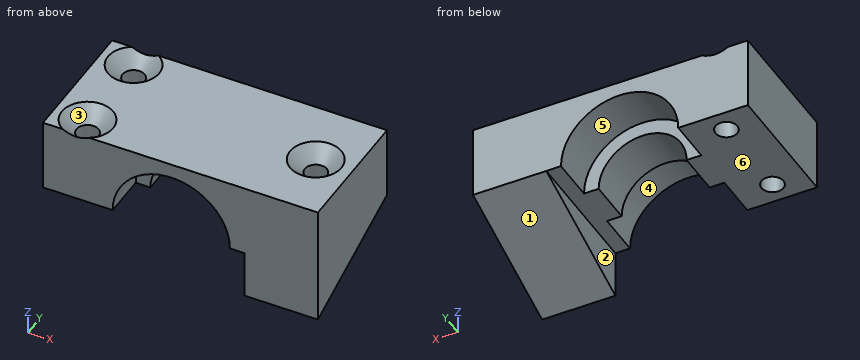
Autodesk Inventor part; units mm, degrees
ref_plane "YZ Plane" through (0, 0, 0) normal (1, 0, 0) x (0, 1, 0)
ref_plane "XZ Plane" through (0, 0, 0) normal (0, 1, 0) x (-1, 0, 0)
ref_plane "XY Plane" through (0, 0, 0) normal (0, 0, 1) x (1, 0, 0)
sketch "Sketch1" plane through (0, 0, 0) normal (0, 0, 1) x (1, 0, 0)
  line L0 (-13.216, 7.0679) -> (17.784, 7.0679) construction
  line L1 (17.784, 7.0679) -> (17.784, -7.9321) construction
  line L2 (17.784, -7.9321) -> (-13.216, -7.9321) construction
  line L3 (-13.216, -7.9321) -> (-13.216, 7.0679) construction
  circle A0 centre (-11.716, 5.5679) radius 1.5
  circle A1 centre (-11.716, -6.4321) radius 1.5
  circle A2 centre (16.284, -0.4321) radius 1.5
  line L4 (-16.216, 8.5679) -> (21.284, 8.5679)
  line L5 (21.284, 8.5679) -> (21.284, -9.4321)
  line L6 (21.284, -9.4321) -> (-16.216, -9.4321)
  line L7 (-16.216, -9.4321) -> (-16.216, 8.5679)
  point P0 (0, 0)
  dimension "d0" = 28
  dimension "d1" = 6
  dimension "d2" = 6
  dimension "d3" = 3
  dimension "d4" = 3
  dimension "d5" = 3
  dimension "d10" = 4.5
  dimension "d11" = 3
  dimension "d13" = 1.5
  dimension "d34" = 5
extrude "Extrusion1" add sketch "Sketch1" along normal blind 10
sketch "Sketch3" plane through (-16.216, -9.4321, 10) normal (0, -1, 0) x (1, 0, 0)
  line L0 (37.5, -10) -> (0, -10)
  circle A0 centre (17.5, -10) radius 6 construction
  line L1 (23.5, -10) -> (23.5, -2.9049) construction
  circle A1 centre (17.5, -10) radius 8
  line L2 (0, -10) -> (0, 0)
  line L3 (9.5, -10) -> (9.5, -3.6397) construction
  point P0 (27.5, -10)
  point P1 (16.216, -10)
  dimension "d19" = 12
  dimension "d21" = 16
  dimension "d30" = 9.5
extrude "Extrusion3" cut sketch "Sketch3" against normal blind 6
sketch "Sketch4" plane through (-16.216, -3.4321, 10) normal (0, -1, 0) x (1, 0, 0)
  arc A0 (25.5, -10) -> (9.5, -10) centre (17.5, -10) ccw
  circle A1 centre (17.5, -10) radius 6
  point P0 (16.216, -10)
  dimension "d24" = 12
extrude "Extrusion4" cut sketch "Sketch4" against normal blind 6
sketch "Sketch5" plane through (-16.216, 2.5679, 10) normal (0, -1, 0) x (1, 0, 0)
  arc A0 (23.5, -10) -> (11.5, -10) centre (17.5, -10) ccw
  circle A1 centre (17.5, -10) radius 8
  point P0 (16.216, -10)
  dimension "d27" = 16
extrude "Extrusion5" cut sketch "Sketch5" against normal blind 19.5
sketch "Sketch6" plane through (21.284, -9.4321, 0) normal (1, 0, 0) x (0, 0, -1)
  line L0 (0, 18) -> (0, 0)
  line L1 (0, 18) -> (-10, 18)
  line L2 (0, 0) -> (-10, 0)
  line L3 (0, 18) -> (6.5515, 0)
  line L4 (0, 18) -> (12.9005, 18) construction
  line L5 (0, 0) -> (6.5515, 0)
  point P0 (0, 9.4321)
  dimension "d31" = 70
extrude "Extrusion6" add sketch "Sketch6" against normal blind 10
chamfer "Chamfer1" distance 2 angle 45 3 edges at (-13.216, 5.5679, 10) (-13.216, -6.4321, 10) (14.784, -0.4321, 10)
equation "\"d4\" = d3"
equation "\"d5\" = d3"
properties part number "Lukker" material "PLA Plastic"
Can you work these out from the model? Positions are in its coordinate system, mm. Face numbers are marked on the shaded views. A direction names the side the tool comes from. Give positions to 0.01 mm unless a question says otherwise; leave off trailing zeros. Order: outer loops, then holes, each group sorted by start corner. A loop starts at its lowest first (then second) coordinate and runs counter-clockwise, first axis right, second up. Notation, with made-up numbers: M 53.25,69 L 102.25,69 A26 ccw 102.25,89 Z; hole C -12.75,21 d4. An arc over 180 degrees is marked long. Use a Markdown table: item, result. Add a question column.
Item 1: Suppose I cut it at C-C (z = -3.75). List the corners of the cut face in (x, y) for me.
Item 2: If I drill on L1, parallel to X at y = -0.5, z = 6.25; L2, parallel to X at y = -7.75, z = 3.75; L3, parallel to X at y = 0.5, z = -1.25, over which ranges is the centre line in solid material (lowest first)? Write a range as [from, to].
Item 3: For the marked faces 4, 5 and 6, which set-ups out of +Z, -Z, +X, -X, +Y, -Y let a thin tool reach every point of the face, with its end or its side?
Item 4: Will these pins go through, and if not, where does the flat tip stop? pin 1 (10 mm diameter, centred on x = -10, y = -4.5, fed in from -Z); pin 2 (5 mm diameter, centred on x = 16.28, y = -0.43, fed in from +Z); pin 3 (9 mm diameter, centred on x = 2.5, z = 2.5, fed in from -Y).
Item 5: Suppose I cut it at B-B (x = 2.5). List the corners of the cut face in (y, z) for me.
Item 6: Suppose I cut it at D-D (x = -3). List the corners of the cut face in (y, z) for me, then the cut area to 3 significant figures.
Item 7: We'd pull the mould along X, two halves only. Please class the marked faces 1, 2 and 3: +X half, -X half, draft (parallel to the pull), parting line (faces both ways), or undercut.
Item 8: Suppose I cut it at A-A (z = 2). List the corners of the cut face in (x, y) for me.
Answer sheet:
| question | item | result |
|---|---|---|
| 1 | outline | M 11.28,-9.43 L 21.28,-9.43 L 21.28,-1.74 L 11.28,-1.74 Z |
| 2 | L1 | x = [-16.22, 14.79], [17.78, 21.28] |
| 2 | L2 | x = [-16.22, -12.43], [-11, -5.78], [8.35, 21.28] |
| 2 | L3 | x = [11.28, 21.28] |
| 3 | face 4 | -Z, -Y |
| 3 | face 5 | -Z, +Y |
| 3 | face 6 | -Z, -X, +Y, -Y |
| 4 | pin 1 | stops at z = 0 |
| 4 | pin 2 | stops at z = 9 |
| 4 | pin 3 | stops at y = -3.43 |
| 5 | outline | M -9.43,7.91 L -3.43,7.91 L -3.43,5.88 L 2.57,5.88 L 2.57,7.91 L 8.57,7.91 L 8.57,10 L -9.43,10 Z |
| 6 | outline | M -9.43,6.76 L -3.43,6.76 L -3.43,4.2 L 2.57,4.2 L 2.57,6.76 L 8.57,6.76 L 8.57,10 L -9.43,10 Z |
| 6 | area | 73.7 mm² |
| 7 | face 1 | draft |
| 7 | face 2 | -X half |
| 7 | face 3 | undercut |
| 8 | outline | M -16.22,-9.43 L -6.46,-9.43 L -6.46,-3.43 L -4.37,-3.43 L -4.37,2.57 L -6.46,2.57 L -6.46,8.57 L -16.22,8.57 Z; M 6.94,-3.43 L 9.03,-3.43 L 9.03,-9.43 L 21.28,-9.43 L 21.28,8.57 L 9.03,8.57 L 9.03,2.57 L 6.94,2.57 Z; hole C -11.72,-6.43 d3; hole C -11.72,5.57 d3; hole C 16.28,-0.43 d3 |
